Build history of the part. All positions in model axes, mm. A direction names the side the tool comes from. Round coordinates to 2 decimals unless told otherwise and drop trailing zeros. Write each loop counter-clockwise with the first axis right and the second up, starting at its lowest first coordinate (ties: lowest second). Pieces come first, ordered by that corner, then holes.
Item 1: 3-axis set-ups, long thin cutter, end or side, ignore diameter. For faces 1 (the cylindrical face through (32.614, -8.872, 28.347)), 2 (the flat face through (81, -8.4, 6.6)), 3 (the flat face through (85.684, -9.571, -5.423)), 4 (the flat face through (86, 0, -11)), 5 (the flat face through (85.68, -9.48, 5.58)): which of +Z, -Z, +X, -X, +Y, -Y reach the whole face in a straight line?
Item 2: Band-saw the part on B-B, the plane x = 84. Write the cut outline in (y, z).
Item 3: Wall check: probe 1 along Y at (x, z) = (113.3, 0); probe 2 along Z at (x, y) = (81.5, -4); probe 3 along X at (y, z) = (-1, 16). Give the ranges that are in metal, low to high.
Item 4: Band-saw the part on D-D, the plane x = 53.5. Write the cut outline in (y, z), then the cut area to 3 significant figures.
Item 5: Drop flat-ended pins along their axis: pin 1 Ø6 at (x, y) = (31, -3.5) entering from +Z; pin 2 Ø8 at (x, z) = (40.5, 1.5) entering from -Y; pin 3 Ø6 at (x, z) = (56, -9.5) entering from +Y. Give the stop position or say it passes through.
Item 6: Mould opens along Z. For faces 6 (the cylindrical face through (34.42, -1.32, -29.97)), 7 (the flat face through (0, 0, 0)), 8 (the flat face through (111, 0, 0)) say: +Z half, -Z half, draft (parallel to the pull), parting line (faces both ways), or undercut.
Item 7: Band-saw the part on C-C, the plane x = 71. Write the cut outline in (y, z).
```python
from build123d import *

# Parameters (mm, degrees)
ZKOSEN_1_SIZE            = 4
SKICA2_R                 = 10
ODEBRAT_VYSUNUT_M1_DEPTH = 2
P_IDAT_VYSUNUT_M1_DEPTH  = 9.5
SKICA4_R                 = 3
SKICA4_R_2               = 2
P_IDAT_VYSUNUT_M2_DEPTH  = 3
SKICA5_R                 = 8.5
P_IDAT_VYSUNUT_M3_DEPTH  = 9


with BuildPart() as part:
    # Skica1 → Rotovat1 (revolve)
    with BuildSketch(Plane.XY, mode=Mode.PRIVATE) as rotovat1_sk:
        Polygon((0, 0), (0, 30), (64, 30), (64, 10.5), (111, 10.5), (111, 0), align=None)
    revolve(rotovat1_sk.sketch.rotate(Axis((0, 0, 0), (1, 0, 0)), 90), axis=Axis((0, 0, 0), (1, 0, 0)))

    # Zkosení1
    zkosen_1_edges = [part.edges().sort_by_distance(p)[0] for p in [
        (0, 0, -30),
    ]]
    chamfer(zkosen_1_edges, length=ZKOSEN_1_SIZE)

    # Skica2 → Odebrat vysunutím1 (cut)
    with BuildSketch(Plane.XY.offset(30)):
        with Locations((28, 0)):
            Circle(SKICA2_R)
    extrude(amount=-ODEBRAT_VYSUNUT_M1_DEPTH, mode=Mode.SUBTRACT)

    # Skica3 → Přidat vysunutím1 (add)
    with BuildSketch(Plane(origin=(81, 0, 0), x_dir=(0, 0, -1), z_dir=(1, 0, 0))):
        Polygon((0, 12.701705922), (-11, 6.350852961), (-11, -6.350852961), (0, -12.701705922), (11, -6.350852961), (11, 6.350852961), align=None)
    extrude(amount=P_IDAT_VYSUNUT_M1_DEPTH)

    # Skica4 → Přidat vysunutím2 (add)
    with BuildSketch(Plane(origin=(111, 0, 0), x_dir=(0, 0, -1), z_dir=(1, 0, 0))):
        with Locations(Location((0, 0, 0), (0, 0, 180))):
            Circle(SKICA4_R)
        Circle(SKICA4_R_2, mode=Mode.SUBTRACT)
    extrude(amount=P_IDAT_VYSUNUT_M2_DEPTH)

    # Skica5 → Přidat vysunutím3 (add)
    with BuildSketch(Plane.XY.offset(28)):
        with Locations((53.5, 0)):
            Circle(SKICA5_R)
    extrude(amount=P_IDAT_VYSUNUT_M3_DEPTH)


solid = part.part
```
Results:
1. face 1: +Z
1. face 2: none
1. face 3: -Z, +X, -Y
1. face 4: -Z, +X, +Y, -Y
1. face 5: +Z, +X, -Y
2. outline: (-12.7, 0) - (-6.35, -11) - (6.35, -11) - (12.7, 0) - (6.35, 11) - (-6.35, 11) - close
3. probe 1: y = -3 to -2, 2 to 3
3. probe 2: z = -11 to 11
3. probe 3: x = 0 to 64
4. outline: (-8.5, 28.77) arc R30 ccw (long way) to (8.5, 28.77) - (8.5, 37) - (-8.5, 37) - close
4. area: 2,950 mm2
5. pin 1: stops at z = 28
5. pin 2: stops at y = -30
5. pin 3: stops at y = 29.29
6. face 6: parting line
6. face 7: draft
6. face 8: undercut
7. outline: circle Ø21 at (0, 0)
